from build123d import *

# Parameters (mm, degrees)
SM_BASE_FLANGE_1_DEPTH = 104
SKETCH_6_R             = 2.75
CUT_EXTRUDE_1_DEPTH    = 3
SKETCH_7_R             = 2.75
CUT_EXTRUDE_3_DEPTH    = 3
SKETCH_8_R             = 18
CUT_EXTRUDE_4_DEPTH    = 3


# Sheet-metal steps are written as plain solids
with BuildPart() as part:
    # Sketch 1 → 基体-法兰1 (new body)
    with BuildSketch(Plane.XY):
        with BuildLine():
            Line((-70, -35), (-70, -4))
            ThreePointArc((-70, -4), (-68.828427125, -1.171572875), (-66, 0))
            Line((-66, 0), (66, 0))
            ThreePointArc((66, 0), (68.828427125, -1.171572875), (70, -4))
            Line((70, -4), (70, -35))
            Line((70, -35), (67, -35))
            Line((67, -35), (67, -4))
            ThreePointArc((67, -4), (66.707106781, -3.292893219), (66, -3))
            Line((66, -3), (-66, -3))
            ThreePointArc((-66, -3), (-66.707106781, -3.292893219), (-67, -4))
            Line((-67, -4), (-67, -35))
            Line((-67, -35), (-70, -35))
        make_face()
    extrude(amount=SM_BASE_FLANGE_1_DEPTH)

    # 草图6 → 切除-拉伸1 (cut)
    with BuildSketch(Plane(origin=(0, 0, 0), x_dir=(1, 0, 0), z_dir=(0, 1, 0))):
        with Locations(Location((24.5, -52, 0), (0, 0, 270))):
            Circle(SKETCH_6_R)
        with Locations(Location((17.324116139, -69.324116139, 0), (0, 0, 270))):
            Circle(SKETCH_6_R)
        with Locations(Location((-17.324116139, -69.324116139, 0), (0, 0, 270))):
            Circle(SKETCH_6_R)
        with Locations(Location((-24.5, -52, 0), (0, 0, 270))):
            Circle(SKETCH_6_R)
        with Locations(Location((-17.324116139, -34.675883861, 0), (0, 0, 270))):
            Circle(SKETCH_6_R)
        with Locations(Location((17.324116139, -34.675883861, 0), (0, 0, 270))):
            Circle(SKETCH_6_R)
    extrude(amount=-CUT_EXTRUDE_1_DEPTH, mode=Mode.SUBTRACT)

    # 草图7 → 切除-拉伸3 (cut)
    with BuildSketch(Plane.ZY.offset(70)):
        with Locations(Location((38, -29, 0), (0, 0, 270))):
            Circle(SKETCH_7_R)
        with Locations(Location((38, -11, 0), (0, 0, 270))):
            Circle(SKETCH_7_R)
        with Locations(Location((6, -11, 0), (0, 0, 270))):
            Circle(SKETCH_7_R)
        with Locations(Location((6, -29, 0), (0, 0, 270))):
            Circle(SKETCH_7_R)
    cut_extrude_3 = extrude(amount=-CUT_EXTRUDE_3_DEPTH, mode=Mode.SUBTRACT)

    # 镜向2: 切除-拉伸3 across plane
    add(cut_extrude_3.mirror(Plane(origin=(0, 0, 0), x_dir=(0, 0, 1), z_dir=(1, 0, 0))), mode=Mode.SUBTRACT)

    # 草图8 → 切除-拉伸4 (cut)
    with BuildSketch(Plane(origin=(0, 0, 0), x_dir=(1, 0, 0), z_dir=(0, 1, 0))):
        with Locations(Location((0, -52, 0), (0, 0, 270))):
            Circle(SKETCH_8_R)
    extrude(amount=-CUT_EXTRUDE_4_DEPTH, mode=Mode.SUBTRACT)


solid = part.part
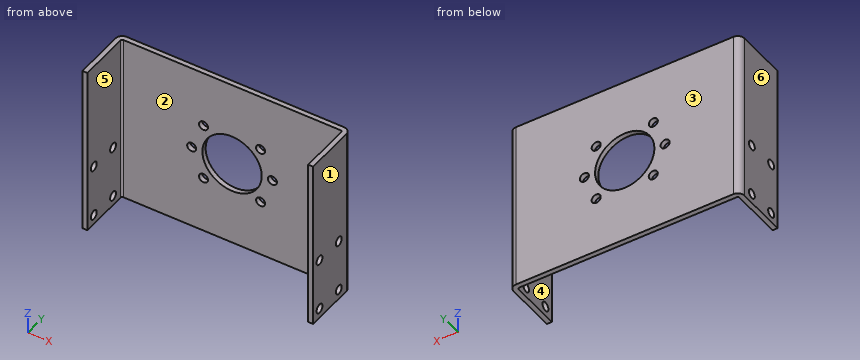
The listing builds one solid part. Answer for the finished solid, in the listing's coordinates (mm). Face numbers are marked on the shaded views. A direction names the side the tool comes from. Coordinates: 2 decimals unless noted, no trailing zeros. Write each loop counter-clockwise with the first axis right and the second up, starting at its lowest first coordinate (ties: lowest second). Pieces come first, ordered by that corner, then holes. Notation, with made-up numbers: (-37.5, 83) - (-25.5, 83) arc R19 ccw to (-25.5, 113) - close; hole circle Ø4 at (-2, 60). An arc over 180 degrees is marked (long way). Return JSON: item names as keys, results as strings.
1. For a pull along X with two mould halves and no side action, classify the marked faces 1, 2, 3 and 4 as +X half, -X half, draft (parallel to the pull), parting line (faces both ways), or undercut.
Final values:
{"face 1": "+X half", "face 2": "undercut", "face 3": "draft", "face 4": "undercut"}
2. Consider line 1 along X through (y, z) = (-4.5, 83); line 2 along Y through (x, z) = (1, 22.5); line 3 along Z through (x, y) = (24, -1). Determine where each line is inside the solid, lowest interval first.
Final values:
{"line 1": "-70 to -67, 67 to 70", "line 2": "-3 to 0", "line 3": "0 to 49.3, 54.7 to 104"}
3. The part is cut by section B-B on y = -18.5. Determine the outline of the cut face in (x, z).
Final values:
{"outline": "(-70, 0) - (-67, 0) - (-67, 104) - (-70, 104) - close; (67, 0) - (70, 0) - (70, 104) - (67, 104) - close"}
4. Each of these flat-tipped pins is pushed along its axis until it touches: pin 1 Ø4.5 at (x, z) = (24.5, 52) entering from -Y; pin 2 Ø7 at (x, z) = (17.32, 34.68) entering from -Y. Where does it stop, or does it pass through?
Final values:
{"pin 1": "through", "pin 2": "y = -3"}
5. The part is cut by section C-C on z = 58. Determine the outline of the cut face in (x, y).
Final values:
{"outline": "(-70, -35) - (-67, -35) - (-67, -4) arc R1 cw to (-66, -3) - (-16.97, -3) - (-16.97, 0) - (-66, 0) arc R4 ccw to (-70, -4) - close; (16.97, -3) - (66, -3) arc R1 cw to (67, -4) - (67, -35) - (70, -35) - (70, -4) arc R4 ccw to (66, 0) - (16.97, 0) - close"}
6. The part is cut by section A-A on x = -24.5. Determine the outline of the cut face in (y, z).
Final values:
{"outline": "(-3, 0) - (0, 0) - (0, 49.25) - (-3, 49.25) - close; (-3, 54.75) - (0, 54.75) - (0, 104) - (-3, 104) - close"}
7. The part is cut by section D-D on y = -29. Determine the outline of the cut face in (x, z), then the cut area to 3 significant figures.
Final values:
{"outline": "(-70, 0) - (-67, 0) - (-67, 3.25) - (-70, 3.25) - close; (-70, 8.75) - (-67, 8.75) - (-67, 35.25) - (-70, 35.25) - close; (-70, 40.75) - (-67, 40.75) - (-67, 104) - (-70, 104) - close; (67, 0) - (70, 0) - (70, 3.25) - (67, 3.25) - close; (67, 8.75) - (70, 8.75) - (70, 35.25) - (67, 35.25) - close; (67, 40.75) - (70, 40.75) - (70, 104) - (67, 104) - close", "area": "558 mm^2"}
8. Which of the six approach directions +Z, -Z, +X, -X, +Y, -Y give full straight-line access (tool end or side, diameter ignored) to the marked faces 5 and 6?
Final values:
{"face 5": "+Z, -Z, -Y", "face 6": "+Z, -Z, -X, +Y, -Y"}
